Geometry check sheet. Reference: the model listing, model coordinates, mm. Face numbers are marked on the shaded views. A direction names the side the tool comes from. Round coordinates to 2 decimals unless told otherwise and drop trailing zeros. Write each loop counter-clockwise with the first axis right and the second up, starting at its lowest first coordinate (ties: lowest second). Pieces come first, ordered by that corner, then holes. Notation, with made-up numbers: M 40.5,50.5 L 52.5,50.5 A12 ccw 52.5,69.5 Z; hole C -24,19 d7. An arc over 180 degrees is marked long. Answer as CSV lines item,"result". Start each with the question number.
```python
from build123d import *

# Parameters (mm, degrees)
F0_R      = 127
F1_DEPTH  = 9.525
F2_R      = 88.9
F3_DEPTH  = 254
F5_W      = 63.5
F5_H      = 76.2
F6_DEPTH  = 76.2
F7_R      = 6.74624
F8_DEPTH  = 25.4
F9_R      = 12.7
F10_R     = 90.17
F10_R_2   = 86.995
F11_DEPTH = 5.08
F12_R     = 8.001
F13_DEPTH = 38.1


with BuildPart() as f1:
    # F0 (on Front) → F1 (new body)
    with BuildSketch(Plane.XZ):
        Circle(F0_R)
    extrude(amount=-F1_DEPTH)

    # F2 (on face) → F3 (join)
    with BuildSketch(Plane(origin=(0, 9.525, 0), x_dir=(-1, 0, 0), z_dir=(0, 1, 0))):
        with Locations((0, -4.739449)):
            Circle(F2_R)
    extrude(amount=F3_DEPTH)

    # F5 (on offset) → F6 (join)
    with BuildSketch(Plane.XY.offset(127)):
        with Locations((0, 184.363604)):
            Rectangle(F5_W, F5_H)
    extrude(amount=-F6_DEPTH)

    # F7 (on face) → F8 (cut)
    with BuildSketch(Plane.XZ):
        with Locations((107.95, 0)):
            Circle(F7_R)
        with Locations((0, 107.95)):
            Circle(F7_R)
        with Locations((-107.95, 0)):
            Circle(F7_R)
        with Locations((0, -107.95)):
            Circle(F7_R)
    extrude(amount=-F8_DEPTH, mode=Mode.SUBTRACT)

    # F9
    f9_edges = [f1.edges().sort_by_distance(p)[0] for p in [
        (88.9, 263.525, -4.739449),
    ]]
    fillet(f9_edges, radius=F9_R)

    # F10 (on face) → F11 (join)
    with BuildSketch(Plane.XZ):
        Circle(F10_R)
        Circle(F10_R_2, mode=Mode.SUBTRACT)
    extrude(amount=F11_DEPTH)

    # F12 (on face) → F13 (join)
    with BuildSketch(Plane.XZ):
        Circle(F12_R)
    extrude(amount=F13_DEPTH)


solid = f1.part
```
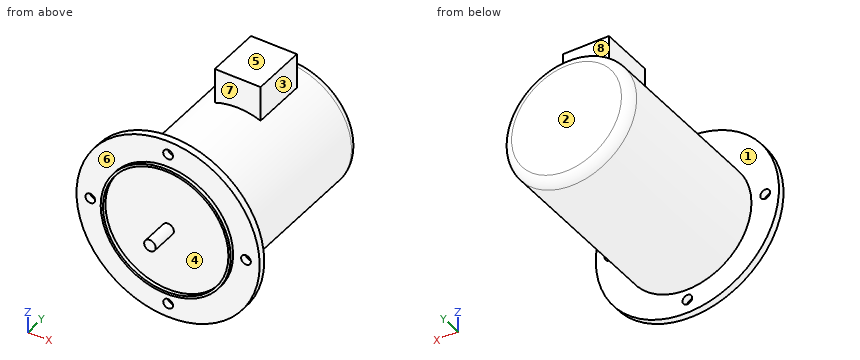
1) Scan lines: line 1 (Y direction, x = -31, z = 114) (3 decimals); line 2 (X direction, y = 245, z = -8.5); line 3 (Z direction, x = -107, y = 2). Record each from-to range of solid material in increasing order. Write a range as from..to.
2) Access from +Z, -Z, +X, -X, +Y, -Y to the whole of each face (thin tool, end or side, straight path). Record for the marked faces 1, 2, 3 and 4.
3) Go/stop test with flat-tipped pins: pin 1 (24.5 mm diameter, centred on x = -11, z = 98.5, fed in from -Y); pin 2 (24.5 mm diameter, centred on x = -0.5, z = 100, fed in from +Y); pin 3 (5 mm diameter, centred on x = 80, y = 184, fed in from +Z). Record where each tip stops, or that it passes through.
4) Section check D-D, the plane z = 107.95. Record the cut outline in (x, y) (3 decimals), plus the area to 3 significant figures.
5) Section check A-A, the plane x = 0. Give the number of separate pieces and of enclosed holes in the cut face, plus the area to 3 significant figures.
6) Section check C-C, the plane x = 107.95. Record the cut outline in (y, z) (3 decimals), plus the area to 3 significant figures.
7) Section check B-B, the plane z = -107.95. Record the cut outline in (x, y) (3 decimals), plus the area to 3 significant figures.
8) Mould release check, pull along Y, two halves, no side actions. Record for the marked faces 5, 6, 7 and 8: released by +Y, released by -Y, zero draft, split by the parting line, or undercut.
Results:
1,line 1,"y = 0..9.525, 146.264..222.464"
1,line 2,"x = -88.82..88.82"
1,line 3,"z = -68.41..-6.68, 6.68..68.41"
2,face 1,"none"
2,face 2,"+Z, -Z, +X, -X, +Y"
2,face 3,"+Z, +X, +Y"
2,face 4,"-Y"
3,pin 1,"stops at y = -5.08"
3,pin 2,"stops at y = 222.46"
3,pin 3,"stops at z = 38.81"
4,outline,"M -66.901,0 L -6.746,0 L -6.746,9.525 L -66.901,9.525 Z; M -31.75,146.264 L 31.75,146.264 L 31.75,222.464 L -31.75,222.464 Z; M 6.746,0 L 66.901,0 L 66.901,9.525 L 6.746,9.525 Z"
4,area,"5,980 mm^2"
5,separate pieces,"3"
5,enclosed holes,"0"
5,area,"51,200 mm^2"
6,outline,"M 0,-66.901 L 9.525,-66.901 L 9.525,-6.746 L 0,-6.746 Z; M 0,6.746 L 9.525,6.746 L 9.525,66.901 L 0,66.901 Z"
6,area,"1,150 mm^2"
7,outline,"M -66.901,0 L -6.746,0 L -6.746,9.525 L -66.901,9.525 Z; M 6.746,0 L 66.901,0 L 66.901,9.525 L 6.746,9.525 Z"
7,area,"1,150 mm^2"
8,face 5,"zero draft"
8,face 6,"released by -Y"
8,face 7,"undercut"
8,face 8,"released by +Y"
